from build123d import *

# Parameters (mm, degrees)
SKETCH_1_R          = 7
SKETCH_1_W          = 20
SKETCH_1_H          = 15
EXTRUDE_1_DEPTH     = 2.5
SKETCH_2_W          = 10
SKETCH_2_H          = 35
CUT_EXTRUDE_3_DEPTH = 671.839026891


with BuildPart() as part:
    # 草图1 → 凸台-拉伸1 (new, symmetric)
    with BuildSketch(Plane.XY):
        with BuildLine():
            Line((-250, 290), (-250, 160))
            ThreePointArc((-250, 160), (-247.071067812, 152.928932188), (-240, 150))
            Line((-240, 150), (240, 150))
            ThreePointArc((240, 150), (247.071067812, 152.928932188), (250, 160))
            Line((250, 160), (250, 290))
            ThreePointArc((250, 290), (252.928932188, 297.071067812), (260, 300))
            Line((260, 300), (590, 300))
            ThreePointArc((590, 300), (597.071067812, 297.071067812), (600, 290))
            Line((600, 290), (600, -290))
            ThreePointArc((600, -290), (597.071067812, -297.071067812), (590, -300))
            Line((590, -300), (260, -300))
            ThreePointArc((260, -300), (252.928932188, -297.071067812), (250, -290))
            Line((250, -290), (250, -160))
            ThreePointArc((250, -160), (247.071067812, -152.928932188), (240, -150))
            Line((240, -150), (-240, -150))
            ThreePointArc((-240, -150), (-247.071067812, -152.928932188), (-250, -160))
            Line((-250, -160), (-250, -290))
            ThreePointArc((-250, -290), (-252.928932188, -297.071067812), (-260, -300))
            Line((-260, -300), (-590, -300))
            ThreePointArc((-590, -300), (-597.071067812, -297.071067812), (-600, -290))
            Line((-600, -290), (-600, 290))
            ThreePointArc((-600, 290), (-597.071067812, 297.071067812), (-590, 300))
            Line((-590, 300), (-260, 300))
            ThreePointArc((-260, 300), (-252.928932188, 297.071067812), (-250, 290))
        make_face()
        with Locations((-580, -225)):
            Circle(SKETCH_1_R, mode=Mode.SUBTRACT)
        with Locations(Location((-580, 225, 0), (0, 0, 180))):
            Circle(SKETCH_1_R, mode=Mode.SUBTRACT)
        with Locations((-270, 225)):
            Circle(SKETCH_1_R, mode=Mode.SUBTRACT)
        with Locations(Location((-270, -225, 0), (0, 0, 180))):
            Circle(SKETCH_1_R, mode=Mode.SUBTRACT)
        with Locations((270, -225)):
            Circle(SKETCH_1_R, mode=Mode.SUBTRACT)
        with Locations(Location((580, -225, 0), (0, 0, 180))):
            Circle(SKETCH_1_R, mode=Mode.SUBTRACT)
        with Locations(Location((270, 225, 0), (0, 0, 180))):
            Circle(SKETCH_1_R, mode=Mode.SUBTRACT)
        with Locations((580, 225)):
            Circle(SKETCH_1_R, mode=Mode.SUBTRACT)
        with Locations((-215, -67.5)):
            Rectangle(SKETCH_1_W, SKETCH_1_H, mode=Mode.SUBTRACT)
        with Locations((-215, 92.5)):
            Rectangle(SKETCH_1_W, SKETCH_1_H, mode=Mode.SUBTRACT)
        with Locations((-215, 67.5)):
            Rectangle(SKETCH_1_W, SKETCH_1_H, mode=Mode.SUBTRACT)
        with Locations((-215, -92.5)):
            Rectangle(SKETCH_1_W, SKETCH_1_H, mode=Mode.SUBTRACT)
        with Locations((215, -92.5)):
            Rectangle(SKETCH_1_W, SKETCH_1_H, mode=Mode.SUBTRACT)
        with Locations((215, 67.5)):
            Rectangle(SKETCH_1_W, SKETCH_1_H, mode=Mode.SUBTRACT)
        with Locations((215, 92.5)):
            Rectangle(SKETCH_1_W, SKETCH_1_H, mode=Mode.SUBTRACT)
        with Locations((215, -67.5)):
            Rectangle(SKETCH_1_W, SKETCH_1_H, mode=Mode.SUBTRACT)
    extrude(amount=EXTRUDE_1_DEPTH, both=True)

    # 草图2 → 切除-拉伸3 (cut, through all)
    with BuildSketch(Plane.XY.offset(2.5)):
        with Locations((-575, 262.5)):
            Rectangle(SKETCH_2_W, SKETCH_2_H)
        with Locations((-575, -262.5)):
            Rectangle(SKETCH_2_W, SKETCH_2_H)
        with Locations((575, -262.5)):
            Rectangle(SKETCH_2_W, SKETCH_2_H)
        with Locations((575, 262.5)):
            Rectangle(SKETCH_2_W, SKETCH_2_H)
        with Locations((275, -262.5)):
            Rectangle(SKETCH_2_W, SKETCH_2_H)
        with Locations((275, 262.5)):
            Rectangle(SKETCH_2_W, SKETCH_2_H)
        with Locations((-275, 262.5)):
            Rectangle(SKETCH_2_W, SKETCH_2_H)
        with Locations((-275, -262.5)):
            Rectangle(SKETCH_2_W, SKETCH_2_H)
    extrude(amount=-CUT_EXTRUDE_3_DEPTH, mode=Mode.SUBTRACT)


solid = part.part
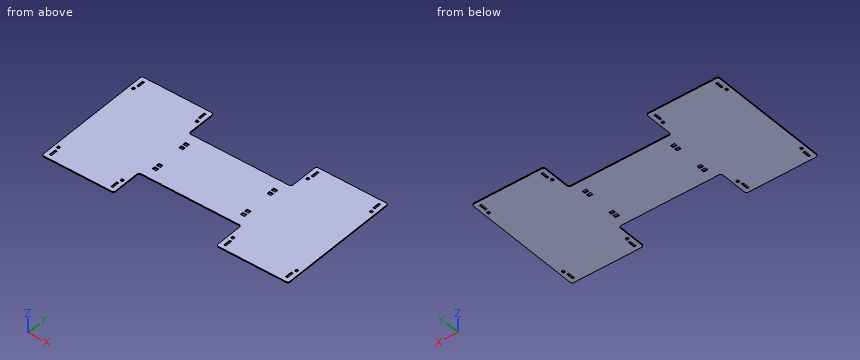
Design review of the part built by this model. Coordinates are the model's own, in mm. Round coordinates to 2 decimals unless told otherwise and drop trailing zeros. Write each loop counter-clockwise with the first axis right and the second up, starting at its lowest first coordinate (ties: lowest second). Pieces come first, ordered by that corner, then holes. Notation, with made-up numbers: M 27,-11.5 L 63,-11.5 A21 ccw 63,-3.5 Z; hole C 61,39 d6. An arc over 180 degrees is marked long. One line per item, written item: value. Start each with the question number.
1. Clearance check with a flat-ended pin moving along its axis: P1, Ø2, axis at x = 37, z = -1, coming from the +Y side. State where the tip first meets the part, or that it passes through.
2. Take a section at A-A on y = 207. State the section outline as (x, z) points.
3. To check wall thickness, follow probe 1 along X at (y, z) = (247, 0.2); probe 2 along X at (y, z) = (-226, -0.45); probe 3 along X at (y, z) = (214.5, -0.5). State the ranges of each line that lie inside material, in increasing order. Write a range as from..to.
4. Take a section at B-B on z = 0.2. State how many separate pieces and enclosed holes the cut face has, then the cut area to 3 significant figures.
5. Take a section at C-C on x = -192. State the section outline as (y, z) points.
Computed:
1. P1: stops at y = 150
2. outline: M -600,-2.5 L -250,-2.5 L -250,2.5 L -600,2.5 Z; M 250,-2.5 L 600,-2.5 L 600,2.5 L 250,2.5 Z
3. probe 1: x = -600..-580, -570..-280, -270..-250, 250..270, 280..570, 580..600
3. probe 2: x = -600..-586.93, -573.07..-276.93, -263.07..-250, 250..263.07, 276.93..573.07, 586.93..600
3. probe 3: x = -600..-250, 250..600
4. separate pieces: 1
4. enclosed holes: 24
4. area: 563,000 mm²
5. outline: M -150,-2.5 L 150,-2.5 L 150,2.5 L -150,2.5 Z
